Read the model definition and answer for the solid it produces. Units are mm, in the model's axes. A direction names the side the tool comes from. Give positions to 0.01 mm unless a question says otherwise; leave off trailing zeros. Order: outer loops, then holes, each group sorted by start corner. A loop starts at its lowest first (then second) coordinate and runs counter-clockwise, first axis right, second up. Notation, with made-up numbers: (63.25, 53.25) - (90.25, 53.25) arc R32 ccw to (90.25, 82.25) - close; hole circle Ø1 at (-32.5, 19.25). An arc over 180 degrees is marked (long way). Return JSON: item names as keys, results as strings.
```python
from build123d import *

# Parameters (mm, degrees)
F1_DEPTH = 431.8
F2_T     = -4.7625
F4_DEPTH = 25.4
F6_DEPTH = 25.4


with BuildPart() as f1:
    # F0 (on Front) → F1 (new body)
    with BuildSketch(Plane.XZ):
        Polygon((273.05, 215.9364468904), (-273.05, 215.9364468904), (-228.6, -152.3635531096), (228.6, -152.3635531096), align=None)
    extrude(amount=F1_DEPTH)

    # F2
    f2_openings = [f1.faces().sort_by_distance(p)[0] for p in [
        (0, -215.9, 215.936447),
    ]]
    offset(amount=F2_T, openings=f2_openings)

    # F3 (on face) → F4 (cut)
    with BuildSketch(Plane(origin=(-243.4427197663, 0, -29.3810179028), x_dir=(0, -1, 0), z_dir=(-0.992795613, 0, -0.1198201602))):
        with BuildLine():
            add(Edge.make_bspline(
                [(152.4, 183.5976519019), (152.4, 139.6035613896), (247.65, 161.6006066457), (342.9, 183.5976519019), (247.65, 205.594697158), (152.4, 227.5917424141), (152.4, 183.5976519019)],
                knots=[0, 0, 0, 2.0943951024, 2.0943951024, 4.1887902048, 4.1887902048, 6.2831853072, 6.2831853072, 6.2831853072], degree=2, weights=[1, 0.5, 1, 0.5, 1, 0.5, 1]))
        make_face()
    extrude(amount=-F4_DEPTH, mode=Mode.SUBTRACT)

    # F5 (on face) → F6 (cut)
    with BuildSketch(Plane(origin=(243.4427197663, 0, -29.3810179028), x_dir=(0, 1, 0), z_dir=(0.992795613, 0, -0.1198201602))):
        with BuildLine():
            add(Edge.make_bspline(
                [(-152.4, 183.5976519019), (-152.4, 227.5917424141), (-247.65, 205.594697158), (-342.9, 183.5976519019), (-247.65, 161.6006066457), (-152.4, 139.6035613896), (-152.4, 183.5976519019)],
                knots=[0, 0, 0, 2.0943951024, 2.0943951024, 4.1887902048, 4.1887902048, 6.2831853072, 6.2831853072, 6.2831853072], degree=2, weights=[1, 0.5, 1, 0.5, 1, 0.5, 1]))
        make_face()
    extrude(amount=-F6_DEPTH, mode=Mode.SUBTRACT)


solid = f1.part
```
Q1. Consider L1, parallel to Y at x = 94.5, z = -10; L2, parallel to Z at x = 204, y = -353; L3, parallel to X at y = -72, z = 77.5. Determine where each line is inside the solid, lowest interval first.
Values:
{"L1": "y = -431.8 to -427.04, -4.76 to 0", "L2": "z = -152.36 to -147.6", "L3": "x = -256.34 to -251.55, 251.55 to 256.34"}
Q2. A cutting plane is placed at A-A (z = 93). Write down the section's boundary in (x, y).
Values:
{"outline": "(-258.21, -431.8) - (258.21, -431.8) - (258.21, 0) - (-258.21, 0) - close; hole (-253.42, -427.04) - (253.42, -427.04) - (253.42, -4.76) - (-253.42, -4.76) - close"}
Q3. A cutting plane is placed at C-C (y = -294). Write down the section's boundary in (x, z), and give its area (3 significant figures).
Values:
{"outline": "(-273.05, 215.94) - (-228.6, -152.36) - (228.6, -152.36) - (273.05, 215.94) - (268.25, 215.94) - (224.38, -147.6) - (-224.38, -147.6) - (-268.25, 215.94) - close", "area": "5,670 mm²"}
Q4. A cutting plane is placed at B-B (x = 98). Write down the section's boundary in (y, z).
Values:
{"outline": "(-431.8, -152.36) - (0, -152.36) - (0, 215.94) - (-4.76, 215.94) - (-4.76, -147.6) - (-427.04, -147.6) - (-427.04, 215.94) - (-431.8, 215.94) - close"}
Q5. Given pin 1 (4 mm diameter, centred on x = -66, y = -240, fed in from +Z); pin 2 (4 mm diameter, centred on y = -211, z = 42.5, fed in from -X); pin 3 (10 mm diameter, centred on y = -384.5, z = -36.5, fed in from +X), each flat-ended and moving along its own axis, determine where each tip first touches the part or whether it passes through.
Values:
{"pin 1": "stops at z = -147.6", "pin 2": "stops at x = -252.36", "pin 3": "stops at x = 243.19"}
Q6. Determine the mould class of faces 3 (the flat face through (-4, 0, 34)), 4 (the flat face through (246.008, -212.944, 31.623)), 5 (the flat face through (-4, -431.8, 34)) for opening direction Y: released by +Y, released by -Y, zero draft, split by the parting line, or undercut.
Values:
{"face 3": "released by +Y", "face 4": "undercut", "face 5": "released by -Y"}
Q7. A cutting plane is placed at D-D (z = 48). Write down the section's boundary in (x, y), and give its area (3 significant figures).
Values:
{"outline": "(-252.78, -431.8) - (252.78, -431.8) - (252.78, 0) - (-252.78, 0) - close; hole (-247.98, -427.04) - (247.98, -427.04) - (247.98, -4.76) - (-247.98, -4.76) - close", "area": "8,870 mm²"}
Q8. For faces 1 (the flat face through (-246.622, -212.944, 36.712)), 2 (the flat face through (-251.136, -212.877, 34.365)), determine the directions among +Z, -Z, +X, -X, +Y, -Y from which every point of the face is accessible in a straight line to the end or side of a thin tool.
Values:
{"face 1": "+Z", "face 2": "-Z, -X, +Y, -Y"}
